Can you work these out from the model? Positions are in its coordinate system, mm. Face numbers are marked on the shaded views. A direction names the side the tool comes from. Coordinates: 2 decimals unless noted, no trailing zeros. Order: outer loops, then holes, each group sorted by start corner. A loop starts at its lowest first (then second) coordinate and runs counter-clockwise, first axis right, second up. Notation, with made-up numbers: (-4.75, 40.25) -> (24.25, 40.25) arc R21 cw to (24.25, 46.25) -> close; hole circle Ø11 at (77, 37). An arc over 180 degrees is marked (long way). Return JSON: item names as keys, results as strings. Group by question number.
1) Thinking about a two-plate mould opening in Y: for the marked faces 4, 5, 6 and 7, which applies, +Y half, -Y half, draft (parallel to the pull), parting line (faces both ways), or undercut?
2) If I drill on probe 1 along Y at (x, z) = (10.75, 8.5); probe 2 along X at (y, z) = (-14, 5); probe 3 along Y at (x, z) = (11.5, 9), over which ranges is the centre line in solid material (lowest first)? Write a range as from..to.
3) For the marked faces 1, 2 and 3, which set-ups out of +Z, -Z, +X, -X, +Y, -Y let a thin tool reach every point of the face, with its end or its side?
4) If we section it at D-D, the plane x = 4.25: Please give me the cut outline in (y, z).
5) If we section it at A-A, the plane z = 1: State how many separate pieces and enclosed holes the cut face has, then the cut area to 3 significant figures.
6) For pin 1 (3 mm diameter, centred on y = -14.5, z = 5.5, fed in from +X); pin 2 (2 mm diameter, centred on y = -25, z = 6.5, fed in from -X); pin 3 (2.5 mm diameter, centred on x = 8.5, y = -19.5, fed in from -Z), each with a flat end and sliding along its axis, tell me the tip position at first contact or that it passes through.
7) If we section it at C-C, the plane y = -16: Please give me the cut outline in (x, z), then the cut area to 3 significant figures.
from build123d import *

# Parameters (mm, degrees)
F0_W     = 5
F0_H     = 10
F1_DEPTH = 10
F2_R     = 1.75
F3_DEPTH = 25
F4_W     = 8
F4_H     = 2
F5_DEPTH = 25
F6_R     = 4.99999
F7_SIZE  = 7
F8_R     = 5


# Not quite as in the source:
# - a fillet or chamfer is up to 0.001 mm smaller than in the source, because OpenCascade refuses the exact size


with BuildPart() as f1:
    # F0 (on Top) → F1 (new body)
    with BuildSketch(Plane.XY):
        Polygon((12, 0), (0, 0), (0, -28), (12, -28), (12, -10), align=None)
        with Locations((14.5, -5)):
            Rectangle(F0_W, F0_H)
    extrude(amount=F1_DEPTH)

    # F2 (on face) → F3 (cut)
    with BuildSketch(Plane.XY.offset(10)):
        with Locations((12, -5)):
            Circle(F2_R)
    extrude(amount=-F3_DEPTH, mode=Mode.SUBTRACT)

    # F4 (on face) → F5 (cut)
    with BuildSketch(Plane(origin=(0, 0, 0), x_dir=(0, -1, 0), z_dir=(-1, 0, 0))):
        with Locations((19, 1)):
            Rectangle(F4_W, F4_H)
        with Locations((19, 9)):
            Rectangle(F4_W, F4_H)
    extrude(amount=-F5_DEPTH, mode=Mode.SUBTRACT)

    # F6 (radius 5 in the source; OpenCascade refuses exactly that, so slightly less here)
    f6_edges = [f1.edges().sort_by_distance(p)[0] for p in [
        (12, -28, 5),
        (0, -28, 5),
        (17, 0, 5),
        (17, -10, 5),
    ]]
    fillet(f6_edges, radius=F6_R)

    # F7
    f7_edges = [f1.edges().sort_by_distance(p)[0] for p in [
        (0, 0, 5),
    ]]
    chamfer(f7_edges, length=F7_SIZE)

    # F8
    f8_edges = [f1.edges().sort_by_distance(p)[0] for p in [
        (7, 0, 5),
        (0, -7, 5),
    ]]
    fillet(f8_edges, radius=F8_R)


solid = f1.part
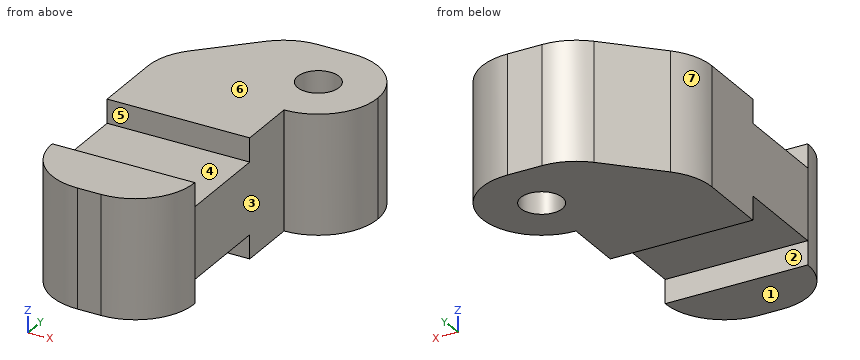
Result sheet:
{
 "1": {"face 4": "undercut", "face 5": "undercut", "face 6": "draft", "face 7": "+Y half"},
 "2": {"probe 1": "y = -26.31..-23, -15..-6.22, -3.78..0", "probe 2": "x = 0..12", "probe 3": "y = -25.18..-23, -15..-6.68, -3.32..0"},
 "3": {"face 1": "-Z, +X, -X, +Y, -Y", "face 2": "-Z, +X, -X", "face 3": "+Z, -Z, +X, -Y"},
 "4": {"outline": "(-27.94, 0) -> (-23, 0) -> (-23, 2) -> (-15, 2) -> (-15, 0) -> (-2.75, 0) -> (-2.75, 10) -> (-15, 10) -> (-15, 8) -> (-23, 8) -> (-23, 10) -> (-27.94, 10) -> close"},
 "5": {"separate pieces": "2", "enclosed holes": "1", "area": "233 mm2"},
 "6": {"pin 1": "stops at x = 12", "pin 2": "stops at x = 0.1", "pin 3": "stops at z = 2"},
 "7": {"outline": "(0, 2) -> (12, 2) -> (12, 8) -> (0, 8) -> close", "area": "72.0 mm2"}
}
